CAD build for the part. Positions are in the model's coordinates, mm. Face numbers are marked on the shaded views. A direction names the side the tool comes from. Give positions to 0.01 mm unless a question says otherwise; leave off trailing zeros. Write each loop counter-clockwise with the first axis right and the second up, starting at its lowest first coordinate (ties: lowest second). Pieces come first, ordered by that corner, then holes. Notation, with made-up numbers: (73.25, 46.5) -> (120.25, 46.5) arc R19 ccw to (120.25, 69.5) -> close; hole circle Ø11 at (63, 74). An arc over 180 degrees is marked (long way). Answer in a Markdown table with one row per item. Add a question column.
```python
from build123d import *

# Parameters (mm, degrees)
F0_W     = 140
F0_H     = 40.4
F1_DEPTH = 1
F2_W     = 10
F2_H     = 40.4
F3_DEPTH = 11
F4_W     = 140
F4_H     = 43.4
F5_DEPTH = 1


with BuildPart() as f1:
    # F0 (on Top) → F1 (new body)
    with BuildSketch(Plane.XY):
        Rectangle(F0_W, F0_H)
    extrude(amount=F1_DEPTH)

    # F2 (on face) → F3 (join)
    with BuildSketch(Plane.XY.offset(1)):
        with Locations((-65, 0)):
            Rectangle(F2_W, F2_H)
        with Locations((65, 0)):
            Rectangle(F2_W, F2_H)
    extrude(amount=F3_DEPTH)

    # F4 (on face) → F5 (join)
    with BuildSketch(Plane(origin=(0, 0, 0), x_dir=(1, 0, 0), z_dir=(0, 0, -1))):
        Rectangle(F4_W, F4_H)
    extrude(amount=F5_DEPTH)


solid = f1.part
```
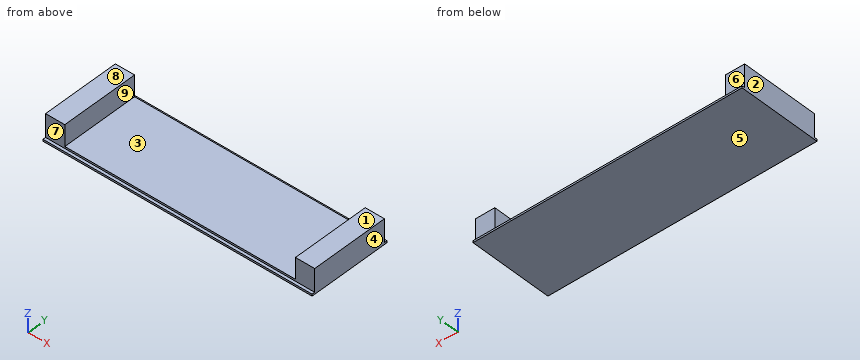
Item 1: Slice it at C-C, the plane y = -2.5. List the corners of the cut face in (x, z).
Item 2: Probe L1, parallel to X at y = -1, z = 6.25; L2, parallel to Y at x = -61.5, z = 8.5; L3, parallel to Z at x = 27.5, y = -4.5. List the from-to ranges inside material, lowest first. Write a range as from..to.
Item 3: Drop flat-ended pins along their axis: pin 1 Ø1.5 at (x, y) = (43.5, 3.5) entering from +Z; pin 2 Ø6 at (x, z) = (-33, 6.5) entering from +Y; pin 3 Ø1.2 at (x, y) = (-6.5, -21) entering from +Z. Give the stop position or say it passes through.
Item 4: Which spindle directions (+Z, -Z, +X, -X, +Y, -Y) get a long thin tool onto all of the face, cutting with end or side? Do the marked faces 5, 6, 7, 8 and 9. Say none if no direction does.
Item 5: Mould opens along X. For the marked faces 1, 2, 3 and 4 say: released by +X, released by -X, zero draft, split by the parting line, or undercut.
Item 6: Slice it at B-B, the plane x = -26.5. List the corners of the cut face in (y, z).
Item 7: Slice it at A-A, the plane z = 4. List the corners of the cut face in (x, y).
Answer key:
| question | item | result |
|---|---|---|
| 1 | outline | (-70, -1) -> (70, -1) -> (70, 12) -> (60, 12) -> (60, 1) -> (-60, 1) -> (-60, 12) -> (-70, 12) -> close |
| 2 | L1 | x = -70..-60, 60..70 |
| 2 | L2 | y = -20.2..20.2 |
| 2 | L3 | z = -1..1 |
| 3 | pin 1 | stops at z = 1 |
| 3 | pin 2 | passes through |
| 3 | pin 3 | stops at z = 0 |
| 4 | face 5 | -Z, +X, -X, +Y, -Y |
| 4 | face 6 | +Z, +X, -X, +Y |
| 4 | face 7 | +Z, +X, -X, -Y |
| 4 | face 8 | +Z, +X, -X, +Y, -Y |
| 4 | face 9 | +Z, +Y, -Y |
| 5 | face 1 | zero draft |
| 5 | face 2 | released by -X |
| 5 | face 3 | undercut |
| 5 | face 4 | released by +X |
| 6 | outline | (-21.7, -1) -> (21.7, -1) -> (21.7, 0) -> (20.2, 0) -> (20.2, 1) -> (-20.2, 1) -> (-20.2, 0) -> (-21.7, 0) -> close |
| 7 | outline | (-70, -20.2) -> (-60, -20.2) -> (-60, 20.2) -> (-70, 20.2) -> close; (60, -20.2) -> (70, -20.2) -> (70, 20.2) -> (60, 20.2) -> close |
